from build123d import *

# Parameters (mm, degrees)
SKETCH1_W           = 110
SKETCH1_H           = 37
SKETCH1_R           = 1.55
BOSS_EXTRUDE1_DEPTH = 5
SKETCH2_W           = 43.75
SKETCH2_H           = 28.75
CUT_EXTRUDE1_DEPTH  = 1.5
SKETCH3_W           = 20
SKETCH3_H           = 35
BOSS_EXTRUDE2_DEPTH = 20
FILLET1_R           = 20
SKETCH4_W           = 7.5
SKETCH4_H           = 7.5
CUT_EXTRUDE2_DEPTH  = 18.75
SKETCH5_W           = 6.5
SKETCH5_H           = 6.5
CUT_EXTRUDE3_DEPTH  = 15
FILLET2_R           = 7.5
CHAMFER1_SIZE       = 0.5
SKETCH7_R           = 4.875
CUT_EXTRUDE5_DEPTH  = 5
SKETCH8_R           = 2.75
CUT_EXTRUDE6_DEPTH  = 2
SKETCH9_W           = 62.5
SKETCH9_H           = 7.5
CUT_EXTRUDE7_DEPTH  = 3
FILLET3_R           = 7.5
FILLET4_R           = 1.5


with BuildPart() as part:
    # Sketch1 → Boss-Extrude1 (new body)
    with BuildSketch(Plane(origin=(0, 0, 0), x_dir=(1, 0, 0), z_dir=(0, 1, 0))):
        Rectangle(SKETCH1_W, SKETCH1_H)
        with Locations(Location((50, -8.5, 0), (0, 0, 270))):
            Circle(SKETCH1_R, mode=Mode.SUBTRACT)
        with Locations(Location((50, 13.5, 0), (0, 0, 270))):
            Circle(SKETCH1_R, mode=Mode.SUBTRACT)
        with Locations(Location((-50, 13.5, 0), (0, 0, 270))):
            Circle(SKETCH1_R, mode=Mode.SUBTRACT)
        with Locations(Location((-50, -8.5, 0), (0, 0, 270))):
            Circle(SKETCH1_R, mode=Mode.SUBTRACT)
    extrude(amount=BOSS_EXTRUDE1_DEPTH)

    # Sketch2 → Cut-Extrude1 (cut)
    with BuildSketch(Plane(origin=(0, 5, 0), x_dir=(1, 0, 0), z_dir=(0, 1, 0))):
        Rectangle(SKETCH2_W, SKETCH2_H)
    extrude(amount=-CUT_EXTRUDE1_DEPTH, mode=Mode.SUBTRACT)

    # Sketch3 → Boss-Extrude2 (add)
    with BuildSketch(Plane(origin=(0, 0, 0), x_dir=(-1, 0, 0), z_dir=(0, -1, 0))):
        with Locations((35, 1)):
            Rectangle(SKETCH3_W, SKETCH3_H)
        with Locations((-35, 1)):
            Rectangle(SKETCH3_W, SKETCH3_H)
    extrude(amount=BOSS_EXTRUDE2_DEPTH)

    # Fillet1
    fillet1_edges = [part.edges().sort_by_distance(p)[0] for p in [
        (35, -20, -18.5),
        (-35, -20, -18.5),
    ]]
    fillet(fillet1_edges, radius=FILLET1_R)

    # Sketch4 → Cut-Extrude2 (cut)
    with BuildSketch(Plane(origin=(0, 5, 0), x_dir=(1, 0, 0), z_dir=(0, 1, 0))):
        with Locations((-35, 0)):
            Rectangle(SKETCH4_W, SKETCH4_H)
        with Locations((35, 0)):
            Rectangle(SKETCH4_W, SKETCH4_H)
    extrude(amount=-CUT_EXTRUDE2_DEPTH, mode=Mode.SUBTRACT)

    # Sketch5 → Cut-Extrude3 (cut)
    with BuildSketch(Plane.XY.offset(16.5)):
        with Locations((-35, -10)):
            Rectangle(SKETCH5_W, SKETCH5_H)
        with Locations((35, -10)):
            Rectangle(SKETCH5_W, SKETCH5_H)
    extrude(amount=-CUT_EXTRUDE3_DEPTH, mode=Mode.SUBTRACT)

    # Fillet2
    fillet2_edges = [part.edges().sort_by_distance(p)[0] for p in [
        (35, -6.75, 3.75),
        (35, -13.75, -3.75),
        (-35, -13.75, -3.75),
        (-35, -6.75, 3.75),
    ]]
    fillet(fillet2_edges, radius=FILLET2_R - 0.0001)  # a hair under: the kernel refuses the full size

    # Chamfer1
    chamfer1_edges = [part.edges().sort_by_distance(p)[0] for p in [
        (-38.25, -6.25005, 3.75),
        (-35, -13.25, 3.75),
        (-31.75, -6.25005, 3.75),
        (31.75, -6.25005, 3.75),
        (35, -13.25, 3.75),
        (38.25, -6.25005, 3.75),
    ]]
    chamfer(chamfer1_edges, length=CHAMFER1_SIZE - 0.0001)  # a hair under: the kernel refuses the full size

    # Sketch7 → Cut-Extrude5 (cut)
    with BuildSketch(Plane.XY.offset(16.5)):
        with Locations((-35, -10)):
            Circle(SKETCH7_R)
        with Locations((35, -10)):
            Circle(SKETCH7_R)
    extrude(amount=-CUT_EXTRUDE5_DEPTH, mode=Mode.SUBTRACT)

    # Sketch8 → Cut-Extrude6 (cut)
    with BuildSketch(Plane.XZ):
        with Locations(Location((-50, 8.5, 0), (0, 0, 270))):
            Circle(SKETCH8_R)
        with Locations(Location((-50, -13.5, 0), (0, 0, 270))):
            Circle(SKETCH8_R)
        with Locations(Location((50, -13.5, 0), (0, 0, 270))):
            Circle(SKETCH8_R)
        with Locations(Location((50, 8.5, 0), (0, 0, 270))):
            Circle(SKETCH8_R)
    extrude(amount=-CUT_EXTRUDE6_DEPTH, mode=Mode.SUBTRACT)

    # Sketch9 → Cut-Extrude7 (cut)
    with BuildSketch(Plane(origin=(0, 5, 0), x_dir=(1, 0, 0), z_dir=(0, 1, 0))):
        Rectangle(SKETCH9_W, SKETCH9_H)
    extrude(amount=-CUT_EXTRUDE7_DEPTH, mode=Mode.SUBTRACT)

    # Fillet3
    fillet3_edges = [part.edges().sort_by_distance(p)[0] for p in [
        (-31.25, 2, 0),
        (31.25, 2, 0),
    ]]
    fillet(fillet3_edges, radius=FILLET3_R)

    # Fillet4
    fillet4_edges = [part.edges().sort_by_distance(p)[0] for p in [
        (-38.75, 5, 0),
        (-30.3125, 5, -3.75),
        (-30.3125, 5, 3.75),
        (38.75, 5, 0),
        (30.3125, 5, 3.75),
        (30.3125, 5, -3.75),
    ]]
    fillet(fillet4_edges, radius=FILLET4_R)


solid = part.part
Input: part model. Units: mm. Frame: model coordinates. A direction names the side the tool comes from. Coordinates: 2 decimals unless noted, no trailing zeros. Write each loop counter-clockwise with the first axis right and the second up, starting at its lowest first coordinate (ties: lowest second). Pieces come first, ordered by that corner, then holes. Notation, with made-up numbers: M 59.25,-35.75 L 109.25,-35.75 A30 cw 109.25,-11.75 Z; hole C -1.5,0.5 d4. An arc over 180 degrees is marked long. Answer as a JSON object with one key per item and string values. Group by question number.
(1) Set-up query: faces 1 (the face through (-31.75, -9, 8)), 2 (the face through (-39, -10, 11.5)), 3 (the face through (-25, -10, -1)), 4 (the face through (31.25, -9, 1)). Return all of +Z, -Z, +X, -X, +Y, -Y with unobstructed straight access to the full face (end or side cutting, diameter ignored); none if empty.
(2) Ray query, line 1 along X through (y, z) = (-10.25, 15.5); line 2 along X through (y, z) = (1.05, 8.5); line 3 along X through (y, z) = (3.15, -13.5). Return the intervals inside material, ascending. Write a range as [from, to].
(3) Contact query for flat-ended pins moving along their axis: P1, Ø6, axis at x = 8, z = -5, coming from the -Y side; P2, Ø3, axis at x = 41, y = -2, coming from the +Z side; P3, Ø6, axis at x = 39.5, z = 3, coming from the +Y side; P4, Ø9, axis at x = 35, y = -10, coming from the -Z side. Output: stop coordinate, or through.
(4) Section A-A on x = -50. Output: boundary loops of the cut face in (y, z), plus the area to 3 significant figures.
(5) Mould query, pull axis X, two halves, no side actions, for faces 5 (the face through (-45, -10, -1)), 6 (the face through (-51, 2, -15)), 7 (the face through (-30, -8, 16.5)). Classes: pulls with the +X half, pulls with the -X half, needs draft (parallel to the pull), parting line crosses it, or undercut.
(6) Section B-B on z = 13. Output: boundary loops of the cut face in (x, y) (3 decimals), plus the area to 3 significant figures.
(7) Section C-C on y = -3.75. Give the number of separate pieces and of enclosed holes in the cut face, plus the area to 3 significant figures.
Result set:
{
 "1": {"face 1": "none", "face 2": "+Z", "face 3": "+Z, -Z, -Y", "face 4": "+Y"},
 "2": {"line 1": "x = [-45, -39.87], [-30.13, -25], [25, 30.13], [39.87, 45]", "line 2": "x = [-55, -52.75], [-47.25, 47.25], [52.75, 55]", "line 3": "x = [-55, -51.55], [-48.45, 48.45], [51.55, 55]"},
 "3": {"P1": "stops at y = 0", "P2": "stops at z = 16.5", "P3": "stops at y = 5", "P4": "stops at z = -17.73"},
 "4": {"outline": "M 0,-18.5 L 5,-18.5 L 5,-15.05 L 2,-15.05 L 2,-16.25 L 0,-16.25 Z; M 0,-10.75 L 2,-10.75 L 2,-11.95 L 5,-11.95 L 5,6.95 L 2,6.95 L 2,5.75 L 0,5.75 Z; M 0,11.25 L 2,11.25 L 2,10.05 L 5,10.05 L 5,18.5 L 0,18.5 Z", "area": "144 mm2"},
 "5": {"face 5": "pulls with the -X half", "face 6": "undercut", "face 7": "needs draft"},
 "6": {"outline": "M -55,0 L -45,0 L -45,-20 L -25,-20 L -25,0 L 25,0 L 25,-20 L 45,-20 L 45,0 L 55,0 L 55,5 L 21.875,5 L 21.875,3.5 L -21.875,3.5 L -21.875,5 L -55,5 Z; hole C -35,-10 d9.75; hole C 35,-10 d9.75", "area": "1,140 mm2"},
 "7": {"separate pieces": "2", "enclosed holes": "2", "area": "1,250 mm2"}
}
